Autodesk Inventor part; units mm, degrees
ref_plane "YZ Plane" through (0, 0, 0) normal (1, 0, 0) x (0, 1, 0)
ref_plane "XZ Plane" through (0, 0, 0) normal (0, 1, 0) x (-1, 0, 0)
ref_plane "XY Plane" through (0, 0, 0) normal (0, 0, 1) x (1, 0, 0)
sketch "Sketch1" plane through (0, 0, 0) normal (0, 1, 0) x (-1, 0, 0)
  circle A0 centre (0, 0) radius 12.7
  dimension "d0" = 25.4
extrude "Extrusion1" add sketch "Sketch1" along normal blind 25.4
hole "Hole1" at (0, 25.4, 0) direction (0, -1, 0) diameter 5.207 end through all counterbore diameter 12.065 counterbore depth 0.762
chamfer "Chamfer1" distance 0.508 angle 45 1 edges at (0, 25.4, -6.0325)
properties part number "Hole Test"
Design review of the part built by this model. Coordinates are the model's own, in mm. A direction names the side the tool comes from. Give positions to 0.01 mm unless a question says otherwise; leave off trailing zeros. Loops run counter-clockwise (first coordinate to the right, second up) from the corner with the lowest first, then second, coordinate; pieces in that order, holes last. Notation, with made-up numbers: M -23.75,11.5 L 16.25,11.5 A21 ccw 16.25,25.5 Z; hole C 39,70 d2. An arc over 180 degrees is marked long. Write item = value, one per line.
Q1. Insertion check: pin 1 (6 mm diameter, centred on x = -3, z = 1.5, fed in from +Y); pin 2 (1.5 mm diameter, centred on y = 9.5, z = -2.5, fed in from -X); pin 3 (5 mm diameter, centred on x = 6, y = 7.5, fed in from +Z). Each pin has a flat end and moves straight along its axis. Give the tip position at first contact, or say it passes through.
Output values:
pin_1 = 25.21
pin_2 = -12.58
pin_3 = 12.21
Q2. We need section B-B (y = 3.75). Give the boundary of the cut face in (x, z).
Output values:
outline = C 0,0 d25.4; hole C 0,0 d5.21
Q3. To check wall thickness, follow line 1 (Z direction, x = 0, y = 14.25); line 2 (Z direction, x = 0, y = 24.75); line 3 (Y direction, x = -2.5, z = -4.75). State the ranges of each line that lie inside material, in increasing order. Write a range as [from, to].
Output values:
line_1 = [-12.7, -2.6], [2.6, 12.7]
line_2 = [-12.7, -6.03], [6.03, 12.7]
line_3 = [0, 24.64]
Q4. We need section D-D (z = -10.5). Give the boundary of the cut face in (x, y), plus the area to 3 significant figures.
Output values:
outline = M -7.14,0 L 7.14,0 L 7.14,25.4 L -7.14,25.4 Z
area = 363 mm^2
Q5. We need section C-C (x = -9). Give the boundary of the cut face in (y, z), plus the area to 3 significant figures.
Output values:
outline = M 0,-8.96 L 25.4,-8.96 L 25.4,8.96 L 0,8.96 Z
area = 455 mm^2
Q6. For faces 1 (the flat face through (1, 24.638, 3)), 2 (the cylindrical face through (-0.782, 12.147, 2.483)), list the 3-axis set-ups (+Z, -Z, +X, -X, +Y, -Y) from which the entire face can be reached by the end or side of a thin tool; tool diameter is ignored.
Output values:
face_1 = +Y
face_2 = +Y, -Y
Q7. We need section A-A (z = 0). Give the boundary of the cut face in (x, y).
Output values:
outline = M -12.7,0 L -2.6,0 L -2.6,24.64 L -6.03,24.64 L -6.03,24.89 L -6.54,25.4 L -12.7,25.4 Z; M 2.6,0 L 12.7,0 L 12.7,25.4 L 6.54,25.4 L 6.03,24.89 L 6.03,24.64 L 2.6,24.64 Z
